Geometry: see drawing. Coordinates: mm, zero at the bounding-box minimum. Give positions to 0.01 mm unless a question says otherwise; leave off trailing zeros. Write each loop counter-clockwise with the first axis right and the second up, starting at its lowest first coordinate (ties: lowest second). Pieces come first, ordered by that corner, then holes. Notation, with made-up numbers: (-20, -8) - (16, -8) arc R21 cw to (16, 3) - close; hole circle Ø7 at (89, -3). An arc over 180 degrees is marked (long way). Return JSON: item names as keys, results as strings.
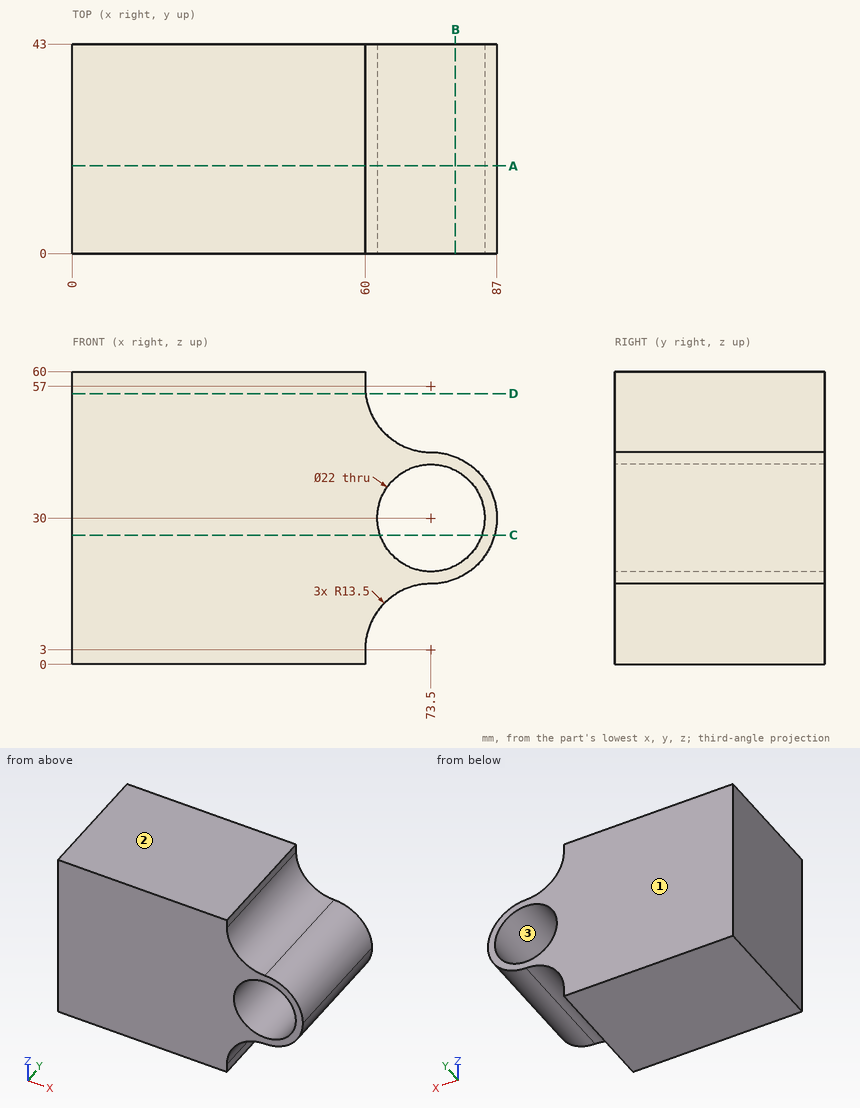
Q1. Section query C-C, the plane z = 26.5. Return the cut outline in (x, y), plus the area to 3 significant figures.
Answer key:
{"outline": "(0, 0) - (63.07, 0) - (63.07, 43) - (0, 43) - close; (83.93, 0) - (86.54, 0) - (86.54, 43) - (83.93, 43) - close", "area": "2,820 mm^2"}
Q2. Pin query (flat end, axial travel): P1, Ø3, axis at x = 59.5, y = 21, coming from the -Z side; P2, Ø0.9, axis at y = 12, z = 1.5, coming from the +X side; P3, Ø12, axis at x = 67, y = 23, coming from the +Z side; P4, Ø10, axis at y = 14.5, z = 44.5, coming from the +X side. Return the tip coordinate at first contact, or that it passes through.
Answer key:
{"P1": "stops at z = 0", "P2": "stops at x = 60", "P3": "stops at z = 51.9", "P4": "stops at x = 83.09"}
Q3. Section query B-B, the plane x = 78.5. Return the cut outline in (y, z).
Answer key:
{"outline": "(0, 17.46) - (43, 17.46) - (43, 20.2) - (0, 20.2) - close; (0, 39.8) - (43, 39.8) - (43, 42.54) - (0, 42.54) - close"}
Q4. Mould query, pull axis Z, two halves, no side actions, for the marked faces 1, 2 and 3. Classes: pulls with the +Z half, pulls with the -Z half, needs draft (parallel to the pull), parting line crosses it, or undercut.
Answer key:
{"face 1": "needs draft", "face 2": "pulls with the +Z half", "face 3": "undercut"}
Q5. Section query D-D, the plane z = 55.5. Return the cut outline in (x, y).
Answer key:
{"outline": "(0, 0) - (60.08, 0) - (60.08, 43) - (0, 43) - close"}
Q6. Section query A-A, the plane y = 18. Return the cut outline in (x, z), plus the area to 3 significant figures.
Answer key:
{"outline": "(0, 0) - (60, 0) - (60, 3) arc R13.5 cw to (73.5, 16.5) arc R13.5 ccw to (73.5, 43.5) arc R13.5 cw to (60, 57) - (60, 60) - (0, 60) - close; hole circle Ø22 at (73.5, 30)", "area": "3,950 mm^2"}
Q7. Material intervals for probe 1 along X at (y, z) = (31, 30); probe 2 along Z at (x, y) = (73, 11); probe 3 along X at (y, z) = (16, 3), sorted ascending. Write a range as [from, to].
Answer key:
{"probe 1": "x = [0, 62.5], [84.5, 87]", "probe 2": "z = [16.49, 19.01], [40.99, 43.51]", "probe 3": "x = [0, 60]"}
